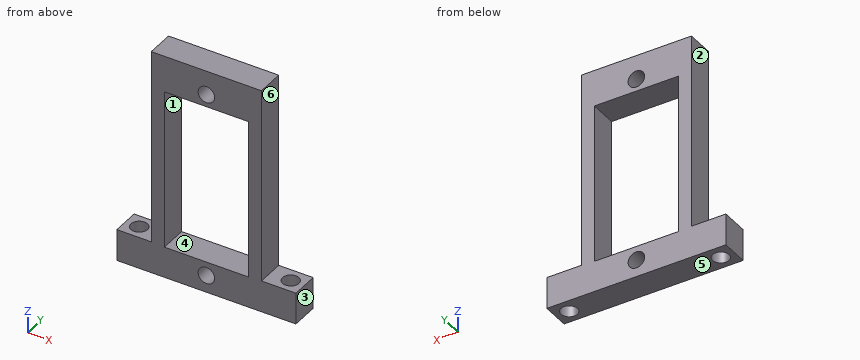
```python
from build123d import *

# Parameters (mm, degrees)
BOX008_W          = 16
BOX008_H          = 4
BOX008_DEPTH      = 33
CYLINDER012_R     = 1.2
CYLINDER012_DEPTH = 20
ARRAY017_X_COUNT  = 2
ARRAY017_X_PITCH  = 22
BOX010_W          = 26
BOX010_H          = 4
BOX010_DEPTH      = 4.6
CYLINDER011_R     = 1.2
CYLINDER011_DEPTH = 4
ARRAY004_Z_COUNT  = 2
ARRAY004_Z_PITCH  = 27
BOX009_W          = 12.2
BOX009_H          = 4
BOX009_DEPTH      = 23.2


with BuildPart() as cube:
    # Box008 → Box008 (new body)
    with BuildSketch(Plane(origin=(-8, 14, 5), x_dir=(1, 0, 0), z_dir=(0, 0, 1))):
        with Locations((8, 2)):
            Rectangle(BOX008_W, BOX008_H)
    extrude(amount=BOX008_DEPTH)


with BuildPart() as connectorscrewcutters:
    # Cylinder012 → Cylinder012 (new body)
    with BuildSketch(Plane(origin=(11, 16, -5), x_dir=(1, 0, 0), z_dir=(0, 0, 1))):
        Circle(CYLINDER012_R)
    extrude(amount=CYLINDER012_DEPTH)

    # Array017 X: ConnectorScrewCutters ×2


with BuildPart() as connectorscrewcutters_1:
    add(connectorscrewcutters.part)
    with Locations(*[(-i * ARRAY017_X_PITCH, 0, 0) for i in range(1, ARRAY017_X_COUNT)]):
        add(connectorscrewcutters.part)


with BuildPart() as cut030:
    # Box010 → Box010 (new body)
    with BuildSketch(Plane(origin=(-13, 14, 5), x_dir=(1, 0, 0), z_dir=(0, 0, 1))):
        with Locations((13, 2)):
            Rectangle(BOX010_W, BOX010_H)
    extrude(amount=BOX010_DEPTH)

    # Cut028: cut ConnectorScrewCutters
    add(connectorscrewcutters_1.part, mode=Mode.SUBTRACT)

    # Cut030: cut Cube
    add(cube.part, mode=Mode.SUBTRACT)


with BuildPart() as screwcutters:
    # Cylinder011 → Cylinder011 (new body)
    with BuildSketch(Plane(origin=(0, 14, 7.5), x_dir=(1, 0, 0), z_dir=(0, 1, 0))):
        Circle(CYLINDER011_R)
    extrude(amount=CYLINDER011_DEPTH)

    # Array004 Z: ScrewCutters ×2


with BuildPart() as screwcutters_1:
    add(screwcutters.part)
    with Locations(*[(0, 0, i * ARRAY004_Z_PITCH) for i in range(1, ARRAY004_Z_COUNT)]):
        add(screwcutters.part)


with BuildPart() as cube001:
    # Box009 → Box009 (new body)
    with BuildSketch(Plane(origin=(-6.1, 14, 9.5), x_dir=(1, 0, 0), z_dir=(0, 0, 1))):
        with Locations((6.1, 2)):
            Rectangle(BOX009_W, BOX009_H)
    extrude(amount=BOX009_DEPTH)


with BuildPart() as cameraconnector:
    # Cut026 base: copy of Cube
    add(cube.part)

    # Cut026: cut Cube001
    add(cube001.part, mode=Mode.SUBTRACT)

    # Cut027: cut ScrewCutters
    add(screwcutters_1.part, mode=Mode.SUBTRACT)

    # Fusion003: union Cut030
    add(cut030.part)


with BuildPart() as cameraconnector_1:
    # Fusion003 placement: moved
    add(cameraconnector.part.moved(Location((0, 0, 485))))


solid = cameraconnector_1.part
```
For this review, take the finished solid that the model builds, in its own axes (mm). Face numbers are marked on the shaded views. A direction names the side the tool comes from. Coordinates: 2 decimals unless noted, no trailing zeros. Write each loop counter-clockwise with the first axis right and the second up, starting at its lowest first coordinate (ties: lowest second). Pieces come first, ordered by that corner, then holes.
(1) Add section C-C on x = 0. Give the boundary of the cut face in (y, z).
(2) Add section D-D on z = 500.5. Give the boundary of the cut face in (x, y).
(3) For pin 1 Ø2 at (y, z) = (16, 509.5) entering from +X; pin 2 Ø1.2 at (y, z) = (16.5, 512) entering from -X; pin 3 Ø2 at (x, y) = (9.5, 16) entering from +Z, all flat-tipped, find the tip position at first contact; note any pin that passes through.
(4) Tool access review of the marked faces 1, 2 and 3: name each direction out of +Z, -Z, +X, -X, +Y, -Y from which nothing blocks a thin tool from reaching the whole face with its end or side.
(5) Add section A-A on y = 16. Give the boundary of the cut face in (x, z).
(6) Add section B-B on z = 492.5. Give the boundary of the cut face in (x, y), then the cut area to 3 significant figures.
(7) The part is to be moulded in two halves that separate along Z. For the marked faces 4, 5 and 6, say which applies: +Z half, -Z half, draft (parallel to the pull), parting line (faces both ways), or undercut.
(8) Wall thickness on probe 1 along Z at (x, y) = (0, 17.25); probe 2 along X at (y, z) = (16, 492.5); probe 3 along Z at (x, y) = (-1.25, 14.5): over which ranges is each line inside the solid? List them lowest first.
Answer sheet:
1. outline: (14, 490) - (18, 490) - (18, 491.3) - (14, 491.3) - close; (14, 493.7) - (18, 493.7) - (18, 494.5) - (14, 494.5) - close; (14, 517.7) - (18, 517.7) - (18, 518.3) - (14, 518.3) - close; (14, 520.7) - (18, 520.7) - (18, 523) - (14, 523) - close
2. outline: (-8, 14) - (-6.1, 14) - (-6.1, 18) - (-8, 18) - close; (6.1, 14) - (8, 14) - (8, 18) - (6.1, 18) - close
3. pin 1: stops at x = 8
3. pin 2: stops at x = -8
3. pin 3: stops at z = 494.6
4. face 1: +Y, -Y
4. face 2: +Z, -X, +Y, -Y
4. face 3: +Z, -Z, +X, +Y, -Y
5. outline: (-13, 490) - (-12.2, 490) - (-12.2, 494.6) - (-13, 494.6) - close; (-9.8, 490) - (9.8, 490) - (9.8, 494.6) - (8, 494.6) - (8, 523) - (-8, 523) - (-8, 494.6) - (-9.8, 494.6) - close; (12.2, 490) - (13, 490) - (13, 494.6) - (12.2, 494.6) - close; hole (-6.1, 494.5) - (6.1, 494.5) - (6.1, 517.7) - (-6.1, 517.7) - close; hole circle Ø2.4 at (0, 492.5); hole circle Ø2.4 at (0, 519.5)
6. outline: (-13, 14) - (-1.2, 14) - (-1.2, 18) - (-13, 18) - close; (1.2, 14) - (13, 14) - (13, 18) - (1.2, 18) - close; hole circle Ø2.4 at (-11, 16); hole circle Ø2.4 at (11, 16)
6. area: 85.4 mm2
7. face 4: undercut
7. face 5: -Z half
7. face 6: draft
8. probe 1: z = 490 to 491.3, 493.7 to 494.5, 517.7 to 518.3, 520.7 to 523
8. probe 2: x = -13 to -12.2, -9.8 to -1.2, 1.2 to 9.8, 12.2 to 13
8. probe 3: z = 490 to 494.5, 517.7 to 523
